Geometry check sheet. Reference: the model listing, model coordinates, mm. A direction names the side the tool comes from. Round coordinates to 2 decimals unless told otherwise and drop trailing zeros. Loops run counter-clockwise (first coordinate to the right, second up) from the corner with the lowest first, then second, coordinate; pieces in that order, holes last.
```python
from build123d import *

# Parameters (mm, degrees)
F0_W     = 34.4444442836
F0_H     = 25
F1_DEPTH = 21.65
F3_D     = 23.3
F5_D     = 2.7
F7_D     = 5.4
F7_DEPTH = 12
F7_TIP   = 1.6223236714


with BuildPart() as f1:
    # F0 (on Top) → F1 (new body)
    with BuildSketch(Plane.XY):
        with Locations((-41.7105928063, 18.1163050001)):
            Rectangle(F0_W, F0_H)
    extrude(amount=F1_DEPTH)

    # F3 (through all)
    with Locations(Plane.XZ.offset(-5.6163050001)):
        with Locations((-41.7105928063, 21.7)):
            Hole(F3_D / 2)

    # F5 (through all)
    with Locations(Plane.XY.offset(21.65)):
        with Locations((-56.1466502289, 26.6163050001), (-56.1466502289, 9.6163050001), (-27.2745353838, 9.6163050001), (-27.2745353838, 26.6163050001)):
            Hole(F5_D / 2)

    # F7
    with Locations(Plane(origin=(0, 0, 0), x_dir=(1, 0, 0), z_dir=(0, 0, -1))):
        with Locations((-56.1466502289, -9.6163050001), (-56.1466502289, -26.6163050001), (-27.2745353838, -26.6163050001), (-27.2745353838, -9.6163050001)):
            Hole(F7_D / 2, depth=F7_DEPTH)
            with Locations((0, 0, -(F7_DEPTH + F7_TIP / 2))):  # 118° drill point
                Cone(0, F7_D / 2, F7_TIP, mode=Mode.SUBTRACT)


solid = f1.part
```
1) Mould release check, pull along Y, two halves, no side actions. Record for faces 1 (the face through (-42, 30.616, 8)), 2 (the face through (-57.434, 10.022, 17.169)), 3 (the face through (-27, 18, 21.65)): +Y half, -Y half, draft (parallel to the pull), parting line (faces both ways), or undercut.
Report:
face 1: +Y half
face 2: undercut
face 3: draft
2) Sectioned sample at B-B, the plane y = 22. Record the cut outline in (x, z).
Report:
outline: (-58.93, 0) - (-24.49, 0) - (-24.49, 21.65) - (-30.06, 21.65) arc R11.65 cw to (-53.36, 21.65) - (-58.93, 21.65) - close
3) Scan lines: line 1 along Y through (x, z) = (-55.5, 5); line 2 along Y through (x, z) = (-27, 2.5); line 3 along X through (y, z) = (27.75, 10) (3 decimals). Record each from-to range of solid material in increasing order.
Report:
line 1: y = 5.62 to 6.99, 12.24 to 23.99, 29.24 to 30.62
line 2: y = 5.62 to 6.93, 12.3 to 23.93, 29.3 to 30.62
line 3: x = -58.933 to -58.597, -53.696 to -29.725, -24.824 to -24.488
4) Sectioned sample at D-D, the plane z = 8.5. Record the cut outline in (x, y), then the cut area to 4 significant figures.
Report:
outline: (-58.93, 5.62) - (-24.49, 5.62) - (-24.49, 30.62) - (-58.93, 30.62) - close; hole circle Ø5.4 at (-56.15, 9.62); hole circle Ø5.4 at (-56.15, 26.62); hole circle Ø5.4 at (-27.27, 9.62); hole circle Ø5.4 at (-27.27, 26.62)
area: 769.5 mm2
5) Gauge pin test, flat ends, axial feed: pin 1 (3 mm diameter, centred on x = -56.15, y = 9.62, fed in from -Z); pin 2 (2 mm diameter, centred on x = -27.27, y = 9.62, fed in from -Z); pin 3 (8 mm diameter, centred on x = -48, y = 13.5, fed in from +Z); pin 4 (2 mm diameter, centred on x = -46, y = 15.5, fed in from +Z). Record the tip position at first contact, or that the pin passes through.
Report:
pin 1: stops at z = 12.72
pin 2: passes through
pin 3: stops at z = 16.24
pin 4: stops at z = 11.32
6) Sectioned sample at A-A, the plane z = 20.25. Record the cut outline in (x, y).
Report:
outline: (-58.93, 5.62) - (-53.27, 5.62) - (-53.27, 30.62) - (-58.93, 30.62) - close; (-30.15, 5.62) - (-24.49, 5.62) - (-24.49, 30.62) - (-30.15, 30.62) - close; hole circle Ø2.7 at (-56.15, 9.62); hole circle Ø2.7 at (-56.15, 26.62); hole circle Ø2.7 at (-27.27, 9.62); hole circle Ø2.7 at (-27.27, 26.62)
7) Sectioned sample at C-C, the plane z = 17. Record the cut outline in (x, y), then the cut area to 3 significant figures.
Report:
outline: (-58.93, 5.62) - (-52.37, 5.62) - (-52.37, 30.62) - (-58.93, 30.62) - close; (-31.05, 5.62) - (-24.49, 5.62) - (-24.49, 30.62) - (-31.05, 30.62) - close; hole circle Ø2.7 at (-56.15, 9.62); hole circle Ø2.7 at (-56.15, 26.62); hole circle Ø2.7 at (-27.27, 9.62); hole circle Ø2.7 at (-27.27, 26.62)
area: 305 mm2
8) Access from +Z, -Z, +X, -X, +Y, -Y to the whole of each face (thin tool, end or side, straight path). Record for faces 4 (the face through (-28.52, 29.01, 6.08)), 5 (the face through (-26.28, 10.53, 17.17)).
Report:
face 4: -Z
face 5: +Z, -Z
